from build123d import *

# Parameters (mm, degrees)
F1_DEPTH = 100


with BuildPart() as f1:
    # F0 (on Top) → F1 (new body)
    with BuildSketch(Plane.XY):
        with BuildLine():
            ThreePointArc((-10.625, 2.420615), (-8.469069, 1.976424), (-7.5, 0))
            ThreePointArc((-7.5, 0), (-8.469069, -1.976424), (-10.625, -2.420615))
            Line((-10.625, -2.420615), (17.5, -9.682458))
            ThreePointArc((17.5, -9.682458), (10, 0), (17.5, 9.682458))
            Line((17.5, 9.682458), (-10.625, 2.420615))
        make_face()
        with BuildLine():
            ThreePointArc((30, 0), (26.123724, 7.905694), (17.5, 9.682458))
            ThreePointArc((17.5, 9.682458), (10, 0), (17.5, -9.682458))
            ThreePointArc((17.5, -9.682458), (26.123724, -7.905694), (30, 0))
        make_face()
        with BuildLine():
            ThreePointArc((-10.625, -2.420615), (-8.469069, -1.976424), (-7.5, 0))
            ThreePointArc((-7.5, 0), (-8.469069, 1.976424), (-10.625, 2.420615))
            ThreePointArc((-10.625, 2.420615), (-12.5, 0), (-10.625, -2.420615))
        make_face()
    extrude(amount=F1_DEPTH)


solid = f1.part
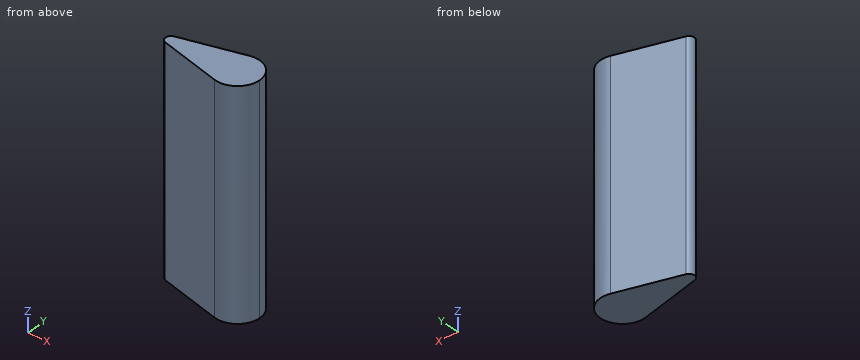
Source: CAD feature listing. Evaluate the final solid. Frame: model axes, mm. Coordinates: 2 decimals unless noted, no trailing zeros. Loops run counter-clockwise (first coordinate to the right, second up) from the corner with the lowest first, then second, coordinate; pieces in that order, holes last. Notation, with made-up numbers: (8, 42.25) - (15, 42.25) arc R36 cw to (15, 79.25) - close; hole circle Ø3 at (-34, 53). An arc over 180 degrees is marked (long way). One line per question, with ' | ' between items.
1) Section A-A, the plane z = 8. Return loops of the section in (x, y) (3 decimals), then the cut area to 3 significant figures.
Report:
outline: (-10.625, -2.421) - (17.5, -9.682) arc R10 ccw (long way) to (17.5, 9.682) - (-10.625, 2.421) arc R2.5 ccw to start | area: 554 mm²
2) Section B-B, the plane x = 7. Return loops of the section in (y, z).
Report:
outline: (-6.97, 0) - (6.97, 0) - (6.97, 100) - (-6.97, 100) - close
3) Section C-C, the plane y = -4.75. Return loops of the section in (x, z).
Report:
outline: (-1.6, 0) - (28.8, 0) - (28.8, 100) - (-1.6, 100) - close
4) Line query: line 1 along X through (y, z) = (0.25, 19); line 2 along Y through (x, z) = (25, 46); line 3 along Y through (x, z) = (-6, 40). Output: solid intervals per line, ascending.
Report:
line 1: x = -12.49 to 30 | line 2: y = -8.66 to 8.66 | line 3: y = -3.61 to 3.61
5) First-contact query: P1, Ø8, axis at y = 5, z = 84, coming from the -X side; P2, Ø1.5, axis at x = 7, z = 79.5, coming from the +Y side (3 decimals); P3, Ø8, axis at x = 12.5, z = 43.5, coming from the +Y side. Flat tips, straight axial feed; report the tip coordinate or a pass-through.
Report:
P1: stops at x = -12.29 | P2: stops at y = 7.165 | P3: stops at y = 9.42
